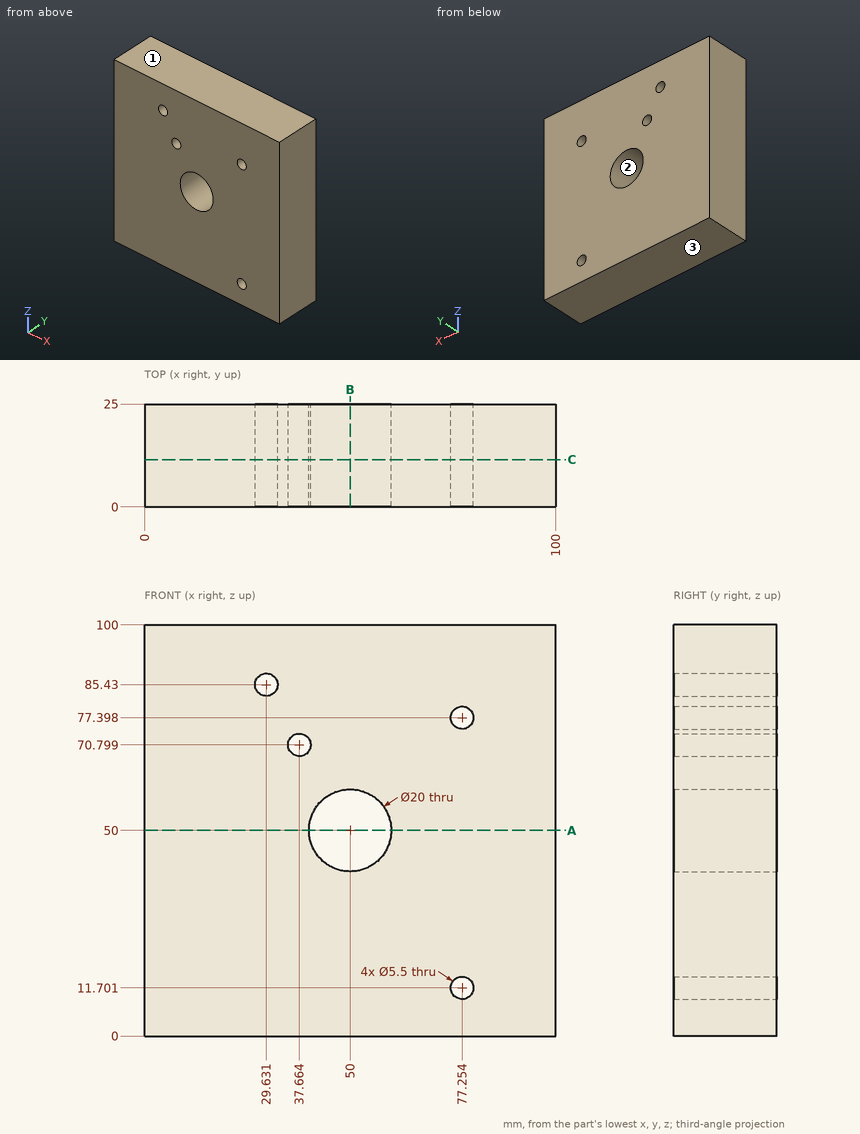
For this review, use the dimensioned drawing (mm, ordinates from the lowest corner) and the shaded views. Round coordinates to 2 decimals unless told otherwise and drop trailing zeros. Write each loop counter-clockwise with the first axis right and the second up, starting at its lowest first coordinate (ties: lowest second). Pieces come first, ordered by that corner, then holes. Notation, with made-up numbers: M 63,87.5 L 118,87.5 A9 ccw 118,103.5 Z; hole C 70,46.5 d2. An arc over 180 degrees is marked long. Use CSV: the item, a comma, the result in double quotes. Start each with the question number.
(1) We need section C-C, the plane y = 11.5. State how many separate pieces and enclosed holes the cut face has, then the cut area to 3 significant figures.
(2) We need section B-B, the plane x = 50. State the section outline as (y, z) points, then the cut area to 3 significant figures.
(3) We need section A-A, the plane z = 50. State the section outline as (x, y) points.
(4) For line 1 along Z through (x, y) = (30, 15.25) (1 decimal); line 2 along Z through (x, y) = (50, 19.75); line 3 along X through (y, z) = (9.25, 70.5), list the stretches that pass through material, from the lowest coordinate up.
(5) Clearance check with a flat-ended pin moving along its axis: P1, Ø4.5, axis at x = 37.66, z = 70.8, coming from the -Y side. State where the tip first meets the part, or that it passes through.
(6) The part is to be moulded in two halves that separate along Z. For the marked faces 1, 2 and 3, say which applies: +Z half, -Z half, draft (parallel to the pull), parting line (faces both ways), or undercut.
Findings:
1,separate pieces,"1"
1,enclosed holes,"5"
1,area,"9,590 mm^2"
2,outline,"M 0,0 L 25,0 L 25,40 L 0,40 Z; M 0,60 L 25,60 L 25,100 L 0,100 Z"
2,area,"2,000 mm^2"
3,outline,"M 0,0 L 40,0 L 40,25 L 0,25 Z; M 60,0 L 100,0 L 100,25 L 60,25 Z"
4,line 1,"0 to 82.7, 88.2 to 100"
4,line 2,"0 to 40, 60 to 100"
4,line 3,"0 to 34.93, 40.4 to 100"
5,P1,"through"
6,face 1,"+Z half"
6,face 2,"undercut"
6,face 3,"-Z half"
